Input: part model. Units: mm. Frame: model coordinates. A direction names the side the tool comes from. Coordinates: 2 decimals unless noted, no trailing zeros. Write each loop counter-clockwise with the first axis right and the second up, starting at its lowest first coordinate (ties: lowest second). Pieces come first, ordered by that corner, then holes. Notation, with made-up numbers: (79.25, -39.5) - (84.25, -39.5) arc R19 ccw to (84.25, -32.5) - close; hole circle Ø5 at (-37.75, -17.75). An arc over 180 degrees is marked (long way). Use a Markdown table: item, result. Add a question column.
Q1. Set-up query: faces 4 (the face through (1, -2, 25.185)), 5 (the face through (5, -2, 44.235)), 6 (the face through (0, -2, -33)). Return all of +Z, -Z, +X, -X, +Y, -Y with unobstructed straight access to the full face (end or side cutting, diameter ignored); none if empty.
Q2. Pin query (flat end, axial travel): P1, Ø1.6, axis at y = -2, z = -36, coming from the +X side; P2, Ø0.8, axis at x = 5.5, y = -2, coming from the -Z side; P3, Ø1.3, axis at x = 1, y = -1, coming from the -Z side. Return the tip coordinate at first contact, or that it passes through.
Q3. Section query A-A (z = -3). Return the cut outline in (x, y) (1 decimal), then the cut area to 3 significant figures.
Q4. Material intervals for probe 1 along Z at (x, y) = (-14.5, -1.2); probe 2 along X at (y, z) = (-0.7, 48.5) (1 decimal); probe 3 along X at (y, z) = (-0.85, -13) (1 decimal), sorted ascending. Write a range as from..to.
Q5. Section query C-C (x = -19.75). Return the cut outline in (y, z) (3 decimals).
Q6. Mould query, pull axis Z, two halves, no side actions, for faces 1 (the face through (7.62, -2, 23)), 2 (the face through (0, -2, -10)), 3 (the face through (5, -2, -31.965)). Classes: released by +Z, released by -Z, zero draft, split by the parting line, or undercut.
Q7. Section query B-B (z = 41). Return the cut outline in (x, y) (1 decimal).
Q8. Section query D-D (y = -1.5). Give the number of separate pieces and of enclosed holes in the cut face, then the cut area to 3 significant figures.
from build123d import *

# Parameters (mm, degrees)
F1_DEPTH = 3.175
F2_R     = 5.08
F3_R     = 5.08
F4_R     = 1.27


with BuildPart() as f1:
    # F0 (on Front) → F1 (new body)
    with BuildSketch(Plane.XZ):
        Polygon((0, 50.585326), (0, 56.935326), (-12.7, 56.935326), (-12.7, -44.664674), (0, -44.664674), (0, -25.614674), (0, -19.264674), (0, -0.192746), (0, 0), (0, 6.135326), (0, 6.157254), (0, 25.185326), (0, 31.535326), align=None)
        Polygon((7.62, 56.935326), (0, 56.935326), (0, 50.585326), (2.54, 50.585326), (2.54, 44.235326), (7.62, 44.235326), align=None)
        Polygon((7.62, 31.535326), (0, 31.535326), (0, 25.185326), (2.54, 25.185326), (2.54, 18.835326), (7.62, 18.835326), align=None)
        Polygon((6.77177, 6.157254), (0, 6.157254), (0, 6.135326), (0, 0), (0, -0.192746), (1.69177, -0.192746), (1.69177, -6.542746), (6.77177, -6.542746), align=None)
        Polygon((0, -19.264674), (0, -25.614674), (2.54, -25.614674), (2.54, -31.964674), (7.62, -31.964674), (7.62, -19.264674), align=None)
        Polygon((-12.7, -44.664674), (-12.7, 56.935326), (-17.4625, 56.935326), (-17.4625, 50.585326), (-14.2875, 50.585326), (-14.2875, 31.535326), (-17.4625, 31.535326), (-17.4625, -0.192746), (-14.2875, -0.192746), (-14.2875, -19.264674), (-17.4625, -19.25371), (-17.4625, -44.664674), align=None)
        Polygon((-17.4625, 50.585326), (-17.4625, 56.935326), (-22.225, 56.935326), (-22.225, -44.664674), (-17.4625, -44.664674), (-17.4625, -19.25371), (-20.637462, -19.242746), (-20.6375, -0.192746), (-17.4625, -0.192746), (-17.4625, 31.535326), (-20.6375, 31.535326), (-20.6375, 50.585326), align=None)
    extrude(amount=F1_DEPTH)

    # F2
    f2_edges = [f1.edges().sort_by_distance(p)[0] for p in [
        (-22.225, -1.5875, 56.935326),
        (-22.225, -1.5875, -44.664674),
        (0, -1.5875, -44.664674),
    ]]
    fillet(f2_edges, radius=F2_R)

    # F3
    f3_edges = [f1.edges().sort_by_distance(p)[0] for p in [
        (7.62, -1.5875, 31.535326),
        (6.77177, -1.5875, 6.157254),
        (7.62, -1.5875, -19.264674),
        (7.62, -1.5875, 56.935326),
    ]]
    fillet(f3_edges, radius=F3_R)

    # F4
    f4_edges = [f1.edges().sort_by_distance(p)[0] for p in [
        (7.62, -1.5875, 18.835326),
        (2.54, -1.5875, 18.835326),
        (6.77177, -1.5875, -6.542746),
        (1.69177, -1.5875, -6.542746),
        (2.54, -1.5875, 44.235326),
        (7.62, -1.5875, 44.235326),
        (7.62, -1.5875, -31.964674),
        (2.54, -1.5875, -31.964674),
    ]]
    fillet(f4_edges, radius=F4_R)


solid = f1.part
Values follow:
| question | item | result |
|---|---|---|
| 1 | face 4 | +Y, -Y |
| 1 | face 5 | +X, +Y, -Y |
| 1 | face 6 | -Z, +Y, -Y |
| 2 | P1 | x = 0 |
| 2 | P2 | z = -31.96 |
| 2 | P3 | z = -25.61 |
| 3 | outline | (-22.2, -3.2) - (-20.6, -3.2) - (-20.6, 0) - (-22.2, 0) - close; (-14.3, -3.2) - (0, -3.2) - (0, 0) - (-14.3, 0) - close; (1.7, -3.2) - (6.8, -3.2) - (6.8, 0) - (1.7, 0) - close |
| 3 | area | 66.5 mm2 |
| 4 | probe 1 | -44.66..-19.26, -0.19..31.54, 50.59..56.94 |
| 4 | probe 2 | -22.2..-20.6, -14.3..0, 2.5..7.6 |
| 4 | probe 3 | -22.2..-20.6, -14.3..0 |
| 5 | outline | (-3.175, -43.946) - (0, -43.946) - (0, -19.246) - (-3.175, -19.246) - close; (-3.175, -0.193) - (0, -0.193) - (0, 31.535) - (-3.175, 31.535) - close; (-3.175, 50.585) - (0, 50.585) - (0, 56.217) - (-3.175, 56.217) - close |
| 6 | face 1 | zero draft |
| 6 | face 2 | undercut |
| 6 | face 3 | released by -Z |
| 7 | outline | (-22.2, -3.2) - (-20.6, -3.2) - (-20.6, 0) - (-22.2, 0) - close; (-14.3, -3.2) - (0, -3.2) - (0, 0) - (-14.3, 0) - close |
| 8 | separate pieces | 1 |
| 8 | enclosed holes | 2 |
| 8 | area | 2,290 mm2 |
